from build123d import *

# Parameters (mm, degrees)
SKETCH1_W           = 110
SKETCH1_H           = 45
BOSS_EXTRUDE1_DEPTH = 115
SHELL1_T            = -2
CUT_EXTRUDE1_REACH  = 167.378
SKETCH2_R           = 16.5
CUT_EXTRUDE2_REACH  = 167.378
SKETCH3_W           = 10
SKETCH3_H           = 10
CUT_EXTRUDE3_REACH  = 167.378
SKETCH4_R           = 4


with BuildPart() as part:
    # Sketch1 → Boss-Extrude1 (new body)
    with BuildSketch(Plane(origin=(0, 0, 0), x_dir=(0, 1, 0), z_dir=(0, 0, 1))):
        with Locations((55, 22.5)):
            Rectangle(SKETCH1_W, SKETCH1_H)
    extrude(amount=BOSS_EXTRUDE1_DEPTH)

    # Shell1
    shell1_openings = [part.faces().sort_by_distance(p)[0] for p in [
        (-22.5, 55, 0),
    ]]
    offset(amount=SHELL1_T, openings=shell1_openings, kind=Kind.INTERSECTION)

    # Sketch2 → Cut-Extrude1 (cut, up to next)
    with BuildSketch(Plane.XZ, mode=Mode.PRIVATE) as cut_extrude1_sk1:
        with Locations(Location((-22.5, 25, 0), (0, 0, 270))):
            Circle(SKETCH2_R)
    cut_extrude1_tool1 = extrude(cut_extrude1_sk1.sketch, amount=-CUT_EXTRUDE1_REACH, mode=Mode.PRIVATE) & part.part
    add(cut_extrude1_tool1.solids().sort_by_distance((-22.5, 0, 25))[0], mode=Mode.SUBTRACT)

    # Sketch3 → Cut-Extrude2 (cut, up to next)
    with BuildSketch(Plane.XY.offset(115), mode=Mode.PRIVATE) as cut_extrude2_sk1:
        with Locations((-22.5, 45)):
            Rectangle(SKETCH3_W, SKETCH3_H)
    cut_extrude2_tool1 = extrude(cut_extrude2_sk1.sketch, amount=-CUT_EXTRUDE2_REACH, mode=Mode.PRIVATE) & part.part
    add(cut_extrude2_tool1.solids().sort_by_distance((-22.5, 45, 115))[0], mode=Mode.SUBTRACT)

    # Sketch4 → Cut-Extrude3 (cut, up to next)
    with BuildSketch(Plane(origin=(0, 110, 0), x_dir=(-1, 0, 0), z_dir=(0, 1, 0)), mode=Mode.PRIVATE) as cut_extrude3_sk1:
        with Locations((22.5, 95)):
            Circle(SKETCH4_R)
    cut_extrude3_tool1 = extrude(cut_extrude3_sk1.sketch, amount=-CUT_EXTRUDE3_REACH, mode=Mode.PRIVATE) & part.part
    add(cut_extrude3_tool1.solids().sort_by_distance((-22.5, 110, 95))[0], mode=Mode.SUBTRACT)


solid = part.part
Design review of the part built by this model. Coordinates are the model's own, in mm. A direction names the side the tool comes from. Round coordinates to 2 decimals unless told otherwise and drop trailing zeros. Write each loop counter-clockwise with the first axis right and the second up, starting at its lowest first coordinate (ties: lowest second). Pieces come first, ordered by that corner, then holes. Notation, with made-up numbers: (35.5, -15) -> (62.5, -15) arc R22 ccw to (62.5, 5) -> close; hole circle Ø7 at (82, 6). An arc over 180 degrees is marked (long way). One line per question, with ' | ' between items.
(1) Draft analysis for pull direction Z (two halves, no side actions). For faces 1 (the cylindrical face through (-28.82, 0.99, 9.76)), 2 (the cylindrical face through (-21.633, 109.014, 91.095)), 3 (the flat face through (-22, 0, 57)), 4 (the flat face through (-23, 54, 115)), state which applies: released by +Z, released by -Z, zero draft, split by the parting line, or undercut.
Result sheet:
face 1: undercut | face 2: undercut | face 3: zero draft | face 4: released by +Z
(2) Take a section at D-D, the plane z = 25. State the section outline as (x, y) points, and give its area (3 significant figures).
Result sheet:
outline: (-45, 0) -> (-39, 0) -> (-39, 2) -> (-43, 2) -> (-43, 108) -> (-2, 108) -> (-2, 2) -> (-6, 2) -> (-6, 0) -> (0, 0) -> (0, 110) -> (-45, 110) -> close | area: 538 mm2
(3) Machinability: for faces 5 (the flat face through (-2, 54, 56)), 6 (the flat face through (-22, 110, 57)), which of the approach directions +Z, -Z, +X, -X, +Y, -Y give a long, thin tool a straight path to every point of the face, cutting with its end or side? Answer none if there is none.
Result sheet:
face 5: -Z | face 6: +Z, -Z, +X, -X, +Y
(4) Take a section at C-C, the plane x = -3.5. State the section outline as (y, z) points, and give its area (3 significant figures).
Result sheet:
outline: (0, 0) -> (2, 0) -> (2, 113) -> (108, 113) -> (108, 0) -> (110, 0) -> (110, 115) -> (0, 115) -> close | area: 672 mm2
(5) Insertion check: P1, Ø0.6, axis at y = 43.5, z = 114, coming from the +X side; P2, Ø6.5, axis at x = -22.5, z = 95, coming from the +Y side; P3, Ø8, axis at x = -17, y = 90.5, coming from the -Z side. Each pin has a flat end and moves straight along its axis. Give the tip position at first contact, or say it passes through.
Result sheet:
P1: x = 0 | P2: y = 2 | P3: z = 113
(6) Take a section at B-B, the plane z = 50.5. State the section outline as (x, y) points.
Result sheet:
outline: (-45, 0) -> (0, 0) -> (0, 110) -> (-45, 110) -> close; hole (-43, 2) -> (-2, 2) -> (-2, 108) -> (-43, 108) -> close
(7) Take a section at A-A, the plane x = -22.5. State the section outline as (y, z) points.
Result sheet:
outline: (0, 0) -> (2, 0) -> (2, 8.5) -> (0, 8.5) -> close; (0, 41.5) -> (2, 41.5) -> (2, 113) -> (40, 113) -> (40, 115) -> (0, 115) -> close; (50, 113) -> (108, 113) -> (108, 99) -> (110, 99) -> (110, 115) -> (50, 115) -> close; (108, 0) -> (110, 0) -> (110, 91) -> (108, 91) -> close
(8) Wall thickness on line 1 (X direction, y = 91.5, z = 60); line 2 (Y direction, x = -41, z = 43); line 3 (Z direction, x = -22.5, y = 108.45): over which ranges is each line inside the solid? List them lowest first. Write a range as [from, to].
Result sheet:
line 1: [-45, -43], [-2, 0] | line 2: [0, 2], [108, 110] | line 3: [0, 91], [99, 115]
